```python
from build123d import *

# Parameters (mm, degrees)
P_IDAT_VYSUNUT_M1_DEPTH   = 12
SKICA2_R                  = 1.75
P_IDAT_VYSUNUT_M1_2_DEPTH = 12
SKICA3_W                  = 38
SKICA3_H                  = 43.5
P_IDAT_VYSUNUT_M2_DEPTH   = 2
P_IDAT_VYSUNUT_M3_DEPTH   = 10.5
SKICA5_W                  = 38
SKICA5_H                  = 5
P_IDAT_VYSUNUT_M4_DEPTH   = 4
SKICA7_W                  = 38
SKICA7_H                  = 76
P_IDAT_VYSUNUT_M5_DEPTH   = 4
SKICA8_W                  = 38
SKICA8_H                  = 42
SKICA8_W_2                = 32
SKICA8_H_2                = 36
P_IDAT_VYSUNUT_M6_DEPTH   = 4
SKICA9_W                  = 35
SKICA9_H                  = 2
ODEBRAT_VYSUNUT_M2_DEPTH  = 40
ODEBRAT_START             = -5
SKICA11_R                 = 1.5
ODEBRAT_VYSUNUT_M3_DEPTH  = 5
P_IDAT_START              = -12
SKICA13_R                 = 1.75
P_IDAT_VYSUNUT_M7_DEPTH   = 12


with BuildPart() as part:
    # Skica2 → P_idat vysunut_m1 (new body)
    with BuildSketch(Plane.XY):
        Polygon((36, 151.5), (36, 114.5), (33, 114.5), (1, 114.5), (-2, 114.5), (-2, 151.5), (-2, 156.5), (36, 156.5), align=None)
        Polygon((33, 151.5), (33, 117.5), (1, 117.5), (1, 151.5), (1, 153.5), (33, 153.5), align=None, mode=Mode.SUBTRACT)
    extrude(amount=P_IDAT_VYSUNUT_M1_DEPTH)



with BuildPart() as body_2:
    # Skica2 → P_idat vysunut_m1 2 (new body)
    with BuildSketch(Plane.XY):
        Polygon((36, -5), (33, -5), (1, -5), (-2, -5), (-2, 71), (1, 71), (33, 71), (36, 71), align=None)
        with Locations((0, -3)):
            Circle(SKICA2_R, mode=Mode.SUBTRACT)
        with Locations((34, -3)):
            Circle(SKICA2_R, mode=Mode.SUBTRACT)
        with BuildLine():
            Line((1, 68), (33, 68))
            Line((33, 68), (33, -1.267949192))
            ThreePointArc((33, -1.267949192), (32.585786438, -1.585786438), (32.267949192, -2))
            Line((32.267949192, -2), (1.732050808, -2))
            ThreePointArc((1.732050808, -2), (1.414213562, -1.585786438), (1, -1.267949192))
            Line((1, -1.267949192), (1, 68))
        make_face(mode=Mode.SUBTRACT)
    extrude(amount=P_IDAT_VYSUNUT_M1_2_DEPTH)


with BuildPart() as part_1:
    add(part.part)

    add(body_2.part)  # P_idat vysunut_m2 merges body 2
    # Skica3 → P_idat vysunut_m2 (add)
    with BuildSketch(Plane.XY):
        with Locations((17, 92.75)):
            Rectangle(SKICA3_W, SKICA3_H)
    extrude(amount=P_IDAT_VYSUNUT_M2_DEPTH)

    # Skica4 → P_idat vysunut_m3 (add)
    with BuildSketch(Plane(origin=(0, 0, 0), x_dir=(-1, 0, 0), z_dir=(0, 0, -1))):
        Polygon((-36, 156.5), (2, 156.5), (2, 154.5), (2, 151.5), (-1, 151.5), (-1, 153.5), (-33, 153.5), (-33, 151.5), (-36, 151.5), (-36, 154.5), align=None)
    extrude(amount=P_IDAT_VYSUNUT_M3_DEPTH)

    # Skica5 → P_idat vysunut_m4 (add)
    with BuildSketch(Plane(origin=(0, 0, -10.5), x_dir=(-1, 0, 0), z_dir=(0, 0, -1))):
        with Locations((-17, 154)):
            Rectangle(SKICA5_W, SKICA5_H)
    extrude(amount=-P_IDAT_VYSUNUT_M4_DEPTH)

    # Skica7 → P_idat vysunut_m5 (add)
    with BuildSketch(Plane.XY.offset(12)):
        with Locations((17, 33)):
            Rectangle(SKICA7_W, SKICA7_H)
    extrude(amount=P_IDAT_VYSUNUT_M5_DEPTH)

    # Skica8 → P_idat vysunut_m6 (add)
    with BuildSketch(Plane.XY.offset(12)):
        with Locations((17, 135.5)):
            Rectangle(SKICA8_W, SKICA8_H)
        with Locations((17, 135.5)):
            Rectangle(SKICA8_W_2, SKICA8_H_2, mode=Mode.SUBTRACT)
    extrude(amount=P_IDAT_VYSUNUT_M6_DEPTH)

    # Skica9 → Odebrat vysunut_m2 (cut)
    with BuildSketch(Plane(origin=(0, 156.5, 0), x_dir=(1, 0, 0), z_dir=(0, 1, 0))):
        with Locations((17, -14)):
            Rectangle(SKICA9_W, SKICA9_H)
    extrude(amount=-ODEBRAT_VYSUNUT_M2_DEPTH, mode=Mode.SUBTRACT)

    # Skica11 → Odebrat vysunut_m3 (cut)
    with BuildSketch(Plane(origin=(0, 156.5, 0), x_dir=(1, 0, 0), z_dir=(0, 1, 0)).offset(ODEBRAT_START)):
        with Locations(Location((0, 8.5, 0), (0, 0, 270))):
            Circle(SKICA11_R)
        with Locations(Location((34, 8.5, 0), (0, 0, 270))):
            Circle(SKICA11_R)
    extrude(amount=ODEBRAT_VYSUNUT_M3_DEPTH, mode=Mode.SUBTRACT)

    # Skica13 → P_idat vysunut_m7 (add)
    with BuildSketch(Plane.XY.offset(16).offset(P_IDAT_START)):
        with Locations((0, -3)):
            Circle(SKICA13_R)
        with Locations((34, -3)):
            Circle(SKICA13_R)
    extrude(amount=P_IDAT_VYSUNUT_M7_DEPTH)


solid = part_1.part
```
Here's how the part is built. I have some questions about the finished solid (model axes, mm). A direction names the side the tool comes from. Give positions to 0.01 mm unless a question says otherwise; leave off trailing zeros. Order: outer loops, then holes, each group sorted by start corner. A loop starts at its lowest first (then second) coordinate and runs counter-clockwise, first axis right, second up. Notation, with made-up numbers: M 40,36 L 54,36 A8 ccw 54,48 Z; hole C -22,16.5 d3. An arc over 180 degrees is marked long. Use a Markdown table: item, result. Add a question column.
1. On a 3-axis mill with a long thin cutter (end or side, diameter ignored), from which of +Z, -Z, +X, -X, +Y, -Y can I reach the whole of each face in a straight line? I mean faces 4 (the flat face through (17, 33, 12)), 5 (the flat face through (17, 153.5, 3)), 6 (the flat face through (17, 117.5, 6)), 7 (the flat face through (17, 154, 15)). Say none if no direction works.
2. I need wall thicknesses on probe 1 along X at (y, z) = (154.3, -8.5); probe 2 along Y at (x, z) = (9, 7); probe 3 along Y at (x, z) = (34, 3.15). Which ranges of each line are inside material? Lowest first, please. Write a range as from..to.
3. Suppose I cut it at C-C (x = 10). List the corners of the cut face in (y, z) for me.
4. If we mould it in two halves opening along X, with no side actions, what happens to faces 1 (the flat face through (17, 151.5, -8)), 2 (the flat face through (33, 34, 6)), 3 (the cylindrical face through (-0.38, -4.71, 1.97))? For each: +X half, -X half, draft (parallel to the pull), parting line (faces both ways), or undercut.
5. Suppose I cut it at D-D (z = -8.5). List the corners of the cut face in (x, y) for me.
6. Suppose I cut it at B-B (y = 131). List the corners of the cut face in (x, z) for me, and give its area (3 significant figures).
7. For pin 1 Ø3.5 at (x, z) = (0, -8.5) entering from +Y; pin 2 Ø3 at (x, z) = (22.5, -6.5) entering from -Y; pin 3 Ø11.5 at (x, y) = (17.5, 62.5) entering from -Z; pin 4 Ø1.6 at (x, z) = (12.5, 14) entering from +Y, each with a flat end and sliding along its axis, tell me the tip position at first contact or that it passes through.
8. Suppose I cut it at A-A (z = 8.75). List the corners of the cut face in (x, y) for me.
Results list:
| question | item | result |
|---|---|---|
| 1 | face 4 | -Z |
| 1 | face 5 | +Z |
| 1 | face 6 | +Z, -Z |
| 1 | face 7 | +Y |
| 2 | probe 1 | x = -2..-1.5, 1.5..32.5, 35.5..36 |
| 2 | probe 2 | y = -5..-2, 68..71, 114.5..117.5, 153.5..156.5 |
| 2 | probe 3 | y = -5..-4.75, -1.25..71, 114.5..156.5 |
| 3 | outline | M -5,0 L -2,0 L -2,12 L 68,12 L 68,0 L 117.5,0 L 117.5,13 L 116.5,13 L 116.5,15 L 117.5,15 L 117.5,16 L 114.5,16 L 114.5,2 L 71,2 L 71,16 L -5,16 Z; M 151.5,-10.5 L 156.5,-10.5 L 156.5,13 L 153.5,13 L 153.5,-6.5 L 151.5,-6.5 Z; M 153.5,15 L 156.5,15 L 156.5,16 L 153.5,16 Z |
| 4 | face 1 | draft |
| 4 | face 2 | undercut |
| 4 | face 3 | undercut |
| 5 | outline | M -2,151.5 L -1.5,151.5 L -1.5,156.5 L -2,156.5 Z; M 1.5,151.5 L 32.5,151.5 L 32.5,156.5 L 1.5,156.5 Z; M 35.5,151.5 L 36,151.5 L 36,156.5 L 35.5,156.5 Z |
| 6 | outline | M -2,0 L 1,0 L 1,13 L -0.5,13 L -0.5,15 L 1,15 L 1,16 L -2,16 Z; M 33,0 L 36,0 L 36,16 L 33,16 L 33,15 L 34.5,15 L 34.5,13 L 33,13 Z |
| 6 | area | 90.0 mm² |
| 7 | pin 1 | stops at y = 156.5 |
| 7 | pin 2 | stops at y = 151.5 |
| 7 | pin 3 | stops at z = 0 |
| 7 | pin 4 | stops at y = 116.5 |
| 8 | outline | M -2,-5 L 36,-5 L 36,71 L -2,71 Z; M -2,114.5 L 36,114.5 L 36,156.5 L -2,156.5 Z; hole M 1,-1.27 A2 cw 1.73,-2 L 32.27,-2 A2 cw 33,-1.27 L 33,68 L 1,68 Z; hole M 1,117.5 L 33,117.5 L 33,153.5 L 1,153.5 Z |
